CAD build for the part. Positions are in the model's coordinates, mm. A direction names the side the tool comes from. Coordinates: 2 decimals unless noted, no trailing zeros. Loops run counter-clockwise (first coordinate to the right, second up) from the corner with the lowest first, then second, coordinate; pieces in that order, holes last. Notation, with made-up numbers: (17.25, 62) -> (39.25, 62) arc R19 cw to (39.25, 98) -> close; hole circle Ø8 at (5.5, 47.25). An arc over 180 degrees is marked (long way). Write each question's results on one line, items separated by ' | '.
```python
from build123d import *

# Parameters (mm, degrees)
F1_DEPTH     = 152.908
F2_R         = 25.4
F3_R         = 1.5875
F4_T1_DEPTH  = 55.1097300731
F4_T3_DEPTH  = 404.8125
F4_T5_DEPTH  = 88.9
F4_T7_DEPTH  = 38.1
F4_T9_DEPTH  = 114.3
F4_T11_DEPTH = 133.8027699269
F4_T14_ANGLE = 90
F4_T16_ANGLE = 90
F4_T18_ANGLE = 90
F4_T20_ANGLE = 90


# Not quite as in the source:
# - a fillet or chamfer that OpenCascade refuses, or shapes differently, is made with other operations: its cross-section is extruded or revolved along the edge and cut away or added


with BuildPart() as f1:
    # F0 (on Top) → F1 (new body)
    with BuildSketch(Plane.XY):
        Polygon((-148.8164286077, -93.2749655156), (-136.1164286077, -93.2749655156), (-136.1164286077, -23.8777354426), (3.5835713923, -23.8777354426), (3.5835713923, 160.7250344844), (-136.1164286077, 160.7250344844), (-136.1164286077, 287.7250344844), (-148.8164286077, 287.7250344844), align=None)
    extrude(amount=F1_DEPTH)

    # F2
    f2_edges = [f1.edges().sort_by_distance(p)[0] for p in [
        (-136.116429, -23.877735, 76.454),
        (3.583571, -23.877735, 76.454),
        (3.583571, 160.725034, 76.454),
        (-136.116429, 160.725034, 76.454),
    ]]
    fillet(f2_edges, radius=F2_R)

    # F3
    f3_edges = [f1.edges().sort_by_distance(p)[0] for p in [
        (-148.816429, -93.274966, 76.454),
        (-136.116429, -93.274966, 76.454),
        (-142.466429, -93.274966, 0),
        (-142.466429, -93.274966, 152.908),
    ]]
    fillet(f3_edges, radius=F3_R)

    # F4: fillet of radius 5.08 on 12 edges, made by hand

    # F4_s2 → F4_t1 (cut)
    with BuildSketch(Plane.XZ.offset(49.2777354426)):
        with BuildLine():
            ThreePointArc((-136.1164286077, 147.828), (-137.6043261593, 151.4201024484), (-141.1964286077, 152.908))
            Line((-141.1964286077, 152.908), (-136.1164286077, 152.908))
            Line((-136.1164286077, 152.908), (-136.1164286077, 147.828))
        make_face()
    extrude(amount=F4_T1_DEPTH, mode=Mode.SUBTRACT)

    # F4_s4 → F4_t3 (cut)
    with BuildSketch(Plane.XZ.offset(-300.4250344844)):
        with BuildLine():
            ThreePointArc((-143.7364286077, 152.908), (-147.3285310561, 151.4201024484), (-148.8164286077, 147.828))
            Line((-148.8164286077, 147.828), (-148.8164286077, 152.908))
            Line((-148.8164286077, 152.908), (-143.7364286077, 152.908))
        make_face()
    extrude(amount=F4_T3_DEPTH, mode=Mode.SUBTRACT)

    # F4_s6 → F4_t5 (cut)
    with BuildSketch(Plane.YZ.offset(-110.7164286077)):
        with BuildLine():
            ThreePointArc((-18.7977354426, 152.908), (-22.389837891, 151.4201024484), (-23.8777354426, 147.828))
            Line((-23.8777354426, 147.828), (-23.8777354426, 152.908))
            Line((-23.8777354426, 152.908), (-18.7977354426, 152.908))
        make_face()
        with BuildLine():
            ThreePointArc((155.6450344844, 152.908), (159.2371369328, 151.4201024484), (160.7250344844, 147.828))
            Line((160.7250344844, 147.828), (160.7250344844, 152.908))
            Line((160.7250344844, 152.908), (155.6450344844, 152.908))
        make_face()
    extrude(amount=F4_T5_DEPTH, mode=Mode.SUBTRACT)

    # F4_s8 → F4_t7 (cut)
    with BuildSketch(Plane.YZ.offset(-161.5164286077)):
        with BuildLine():
            ThreePointArc((282.6450344844, 152.908), (286.2371369328, 151.4201024484), (287.7250344844, 147.828))
            Line((287.7250344844, 147.828), (287.7250344844, 152.908))
            Line((287.7250344844, 152.908), (282.6450344844, 152.908))
        make_face()
    extrude(amount=F4_T7_DEPTH, mode=Mode.SUBTRACT)

    # F4_s10 → F4_t9 (cut)
    with BuildSketch(Plane.XZ.offset(-300.4250344844)):
        with BuildLine():
            ThreePointArc((-141.1964286077, 152.908), (-137.6043261593, 151.4201024484), (-136.1164286077, 147.828))
            Line((-136.1164286077, 147.828), (-136.1164286077, 152.908))
            Line((-136.1164286077, 152.908), (-141.1964286077, 152.908))
        make_face()
    extrude(amount=F4_T9_DEPTH, mode=Mode.SUBTRACT)

    # F4_s12 → F4_t11 (cut)
    with BuildSketch(Plane.XZ.offset(-135.3250344844)):
        with BuildLine():
            ThreePointArc((-1.4964286077, 152.908), (2.0956738407, 151.4201024484), (3.5835713923, 147.828))
            Line((3.5835713923, 147.828), (3.5835713923, 152.908))
            Line((3.5835713923, 152.908), (-1.4964286077, 152.908))
        make_face()
    extrude(amount=F4_T11_DEPTH, mode=Mode.SUBTRACT)

    # F4_s13 → F4_t14 (revolve, cut)
    with BuildSketch(Plane.XZ.offset(49.2777354426)):
        with BuildLine():
            ThreePointArc((-136.1164286077, 147.828), (-137.6043261593, 151.4201024484), (-141.1964286077, 152.908))
            Line((-141.1964286077, 152.908), (-136.1164286077, 152.908))
            Line((-136.1164286077, 152.908), (-136.1164286077, 147.828))
        make_face()
    revolve(axis=Axis((-110.7164286077, -49.2777354426, 152.908), (0, 0, -1)), revolution_arc=F4_T14_ANGLE, mode=Mode.SUBTRACT)

    # F4_s15 → F4_t16 (revolve, cut)
    with BuildSketch(Plane.YZ.offset(-21.8164286077)):
        with BuildLine():
            ThreePointArc((-18.7977354426, 152.908), (-22.389837891, 151.4201024484), (-23.8777354426, 147.828))
            Line((-23.8777354426, 147.828), (-23.8777354426, 152.908))
            Line((-23.8777354426, 152.908), (-18.7977354426, 152.908))
        make_face()
    revolve(axis=Axis((-21.8164286077, 1.5222645574, 152.908), (0, 0, 1)), revolution_arc=F4_T16_ANGLE, mode=Mode.SUBTRACT)

    # F4_s17 → F4_t18 (revolve, cut)
    with BuildSketch(Plane.YZ.offset(-110.7164286077)):
        with BuildLine():
            ThreePointArc((155.6450344844, 152.908), (159.2371369328, 151.4201024484), (160.7250344844, 147.828))
            Line((160.7250344844, 147.828), (160.7250344844, 152.908))
            Line((160.7250344844, 152.908), (155.6450344844, 152.908))
        make_face()
    revolve(axis=Axis((-110.7164286077, 186.1250344844, 152.908), (0, 0, -1)), revolution_arc=F4_T18_ANGLE, mode=Mode.SUBTRACT)

    # F4_s19 → F4_t20 (revolve, cut)
    with BuildSketch(Plane.XZ.offset(-135.3250344844)):
        with BuildLine():
            ThreePointArc((-1.4964286077, 152.908), (2.0956738407, 151.4201024484), (3.5835713923, 147.828))
            Line((3.5835713923, 147.828), (3.5835713923, 152.908))
            Line((3.5835713923, 152.908), (-1.4964286077, 152.908))
        make_face()
    revolve(axis=Axis((-21.8164286077, 135.3250344844, 152.908), (0, 0, 1)), revolution_arc=F4_T20_ANGLE, mode=Mode.SUBTRACT)


solid = f1.part
```
Q1. Which spindle directions (+Z, -Z, +X, -X, +Y, -Y) get a long thin tool onto all of the face, cutting with end or side? Do faces 1 (the flat face through (-67, -23.878, 73)), 2 (the flat face through (-66, 160.725, 73)), 3 (the flat face through (-91, 101, 0)). Say none if no direction does.
Results are:
face 1: +Z, -Z, +X, -Y | face 2: +Z, -Z, +X, +Y | face 3: -Z, +X, -X, +Y, -Y
Q2. Drop flat-ended pins along their axis: pin 1 (1.5 mm diameter, centred on x = -32.5, z = 129, fed in from +Y); pin 2 (12 mm diameter, centred on x = -126, z = 48.5, fed in from +Y); pin 3 (6 mm diameter, centred on x = -33, y = -14.5, fed in from -Z); pin 4 (10 mm diameter, centred on x = -30.5, z = 52.5, fed in from -Y). Give the stop position or say it passes through.
Results are:
pin 1: y = 160.73 | pin 2: y = 172.26 | pin 3: z = 0 | pin 4: y = -23.88
Q3. Wall check: L1, parallel to Y at x = -49, z = 129; L2, parallel to X at y = 240, z = 134.5; L3, parallel to X at y = -0.5, z = 73.5. Give the ranges that are in metal, low to high. Write a range as from..to.
Results are:
L1: -23.88..160.73 | L2: -148.82..-136.12 | L3: -148.82..3.5
Q4. Cut at B-B on y = 198.5. Write the cut outline in (x, z), and give its area (3 significant figures).
Results are:
outline: (-148.82, 0) -> (-136.12, 0) -> (-136.12, 147.83) arc R5.08 ccw to (-141.2, 152.91) -> (-143.74, 152.91) arc R5.08 ccw to (-148.82, 147.83) -> close | area: 1,930 mm^2
Q5. Cut at A-A on x = -39.5. Write the cut outline in (y, z), and give its area (3 significant figures).
Results are:
outline: (-23.88, 0) -> (160.73, 0) -> (160.73, 147.83) arc R5.08 ccw to (155.65, 152.91) -> (-18.8, 152.91) arc R5.08 ccw to (-23.88, 147.83) -> close | area: 28,200 mm^2
Q6. Cut at C-C on z = 75. Write the cut outline in (x, y) (1 decimal).
Results are:
outline: (-148.8, -91.7) arc R1.6 ccw to (-147.2, -93.3) -> (-137.7, -93.3) arc R1.6 ccw to (-136.1, -91.7) -> (-136.1, -49.3) arc R25.4 cw to (-110.7, -23.9) -> (-21.8, -23.9) arc R25.4 ccw to (3.6, 1.5) -> (3.6, 135.3) arc R25.4 ccw to (-21.8, 160.7) -> (-110.7, 160.7) arc R25.4 cw to (-136.1, 186.1) -> (-136.1, 287.7) -> (-148.8, 287.7) -> close
